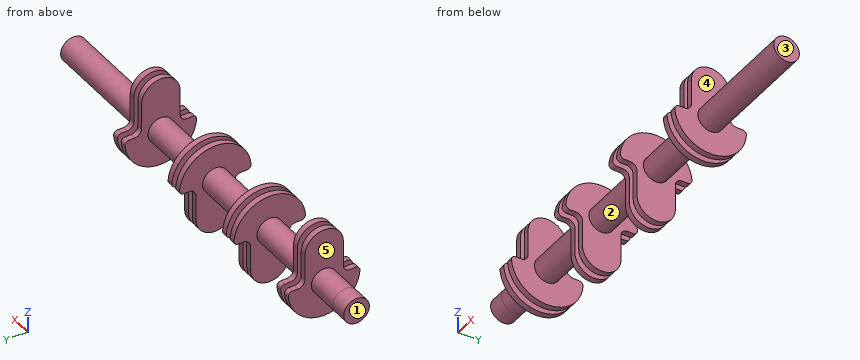
```python
from build123d import *

# Parameters (mm, degrees)
SKETCH1_R               = 15
BOSS_EXTRUDE1_DEPTH     = 400
BOSS_EXTRUDE2_START     = 53.5
BOSS_EXTRUDE2_DEPTH     = 7
BOSS_EXTRUDE3_START     = 39.5
BOSS_EXTRUDE3_DEPTH     = 7
BOSS_EXTRUDE4_START     = 339.5
BOSS_EXTRUDE4_DEPTH     = 7
BOSS_EXTRUDE5_START     = 353.5
BOSS_EXTRUDE5_DEPTH     = 7
CUT_EXTRUDE1_DEPTH      = 60
CUT_EXTRUDE1_DEPTH_BACK = 31
SKETCH5_W               = 7
SKETCH5_H               = 34.934316099
SKETCH5_H_2             = 32.180943616
BOSS_EXTRUDE6_START     = 46.5
SKETCH2_8_R             = 15
BOSS_EXTRUDE6_DEPTH     = 7
BOSS_EXTRUDE7_START     = 346.5
SKETCH2_9_R             = 15
BOSS_EXTRUDE7_DEPTH     = 7
BOSS_EXTRUDE8_START     = 139.5
BOSS_EXTRUDE8_DEPTH     = 7
BOSS_EXTRUDE9_START     = 153.5
BOSS_EXTRUDE9_DEPTH     = 7
BOSS_EXTRUDE10_START    = 239.5
BOSS_EXTRUDE10_DEPTH    = 7
BOSS_EXTRUDE11_START    = 253.5
BOSS_EXTRUDE11_DEPTH    = 7
CUT_EXTRUDE3_DEPTH      = 33
CUT_EXTRUDE3_DEPTH_BACK = 33
SKETCH8_W               = 7
SKETCH8_H               = 30
BOSS_EXTRUDE12_START    = 146.5
SKETCH6_6_R             = 15
BOSS_EXTRUDE12_DEPTH    = 7
BOSS_EXTRUDE13_START    = 246.5
SKETCH6_7_R             = 15
BOSS_EXTRUDE13_DEPTH    = 7
SKETCH9_R               = 15
BOSS_EXTRUDE14_DEPTH    = 100
SKETCH10_R              = 15
BOSS_EXTRUDE15_DEPTH    = 20


with BuildPart() as part:
    # Sketch1 → Boss-Extrude1 (new body)
    with BuildSketch(Plane(origin=(0, 0, 0), x_dir=(0, 0, -1), z_dir=(1, 0, 0))):
        Circle(SKETCH1_R)
    extrude(amount=BOSS_EXTRUDE1_DEPTH)

    # Sketch2 → Boss-Extrude2 (add)
    with BuildSketch(Plane.ZY.offset(-400).offset(BOSS_EXTRUDE2_START)):
        with BuildLine():
            Line((2, 30.5), (2, 37))
            ThreePointArc((2, 37), (0.389660992, 40.675622173), (-3.404079344, 41.983645241))
            ThreePointArc((-3.404079344, 41.983645241), (-42.121422387, 0), (-3.404079344, -41.983645241))
            ThreePointArc((-3.404079344, -41.983645241), (0.389660992, -40.675622173), (2, -37))
            Line((2, -37), (2, -30.5))
            ThreePointArc((2, -30.5), (4.343145751, -24.843145751), (10, -22.5))
            Line((10, -22.5), (40, -22.5))
            ThreePointArc((40, -22.5), (62.5, 0), (40, 22.5))
            Line((40, 22.5), (10, 22.5))
            ThreePointArc((10, 22.5), (4.343145751, 24.843145751), (2, 30.5))
        make_face()
    extrude(amount=BOSS_EXTRUDE2_DEPTH)

    # Sketch2_3 → Boss-Extrude3 (add)
    with BuildSketch(Plane.ZY.offset(-400).offset(BOSS_EXTRUDE3_START)):
        with BuildLine():
            Line((2, 30.5), (2, 37))
            ThreePointArc((2, 37), (0.389660992, 40.675622173), (-3.404079344, 41.983645241))
            ThreePointArc((-3.404079344, 41.983645241), (-42.121422387, 0), (-3.404079344, -41.983645241))
            ThreePointArc((-3.404079344, -41.983645241), (0.389660992, -40.675622173), (2, -37))
            Line((2, -37), (2, -30.5))
            ThreePointArc((2, -30.5), (4.343145751, -24.843145751), (10, -22.5))
            Line((10, -22.5), (40, -22.5))
            ThreePointArc((40, -22.5), (62.5, 0), (40, 22.5))
            Line((40, 22.5), (10, 22.5))
            ThreePointArc((10, 22.5), (4.343145751, 24.843145751), (2, 30.5))
        make_face()
    extrude(amount=BOSS_EXTRUDE3_DEPTH)

    # Sketch2_5 → Boss-Extrude4 (add)
    with BuildSketch(Plane.ZY.offset(-400).offset(BOSS_EXTRUDE4_START)):
        with BuildLine():
            Line((2, 30.5), (2, 37))
            ThreePointArc((2, 37), (0.389660992, 40.675622173), (-3.404079344, 41.983645241))
            ThreePointArc((-3.404079344, 41.983645241), (-42.121422387, 0), (-3.404079344, -41.983645241))
            ThreePointArc((-3.404079344, -41.983645241), (0.389660992, -40.675622173), (2, -37))
            Line((2, -37), (2, -30.5))
            ThreePointArc((2, -30.5), (4.343145751, -24.843145751), (10, -22.5))
            Line((10, -22.5), (40, -22.5))
            ThreePointArc((40, -22.5), (62.5, 0), (40, 22.5))
            Line((40, 22.5), (10, 22.5))
            ThreePointArc((10, 22.5), (4.343145751, 24.843145751), (2, 30.5))
        make_face()
    extrude(amount=BOSS_EXTRUDE4_DEPTH)

    # Sketch2_6 → Boss-Extrude5 (add)
    with BuildSketch(Plane.ZY.offset(-400).offset(BOSS_EXTRUDE5_START)):
        with BuildLine():
            Line((2, 30.5), (2, 37))
            ThreePointArc((2, 37), (0.389660992, 40.675622173), (-3.404079344, 41.983645241))
            ThreePointArc((-3.404079344, 41.983645241), (-42.121422387, 0), (-3.404079344, -41.983645241))
            ThreePointArc((-3.404079344, -41.983645241), (0.389660992, -40.675622173), (2, -37))
            Line((2, -37), (2, -30.5))
            ThreePointArc((2, -30.5), (4.343145751, -24.843145751), (10, -22.5))
            Line((10, -22.5), (40, -22.5))
            ThreePointArc((40, -22.5), (62.5, 0), (40, 22.5))
            Line((40, 22.5), (10, 22.5))
            ThreePointArc((10, 22.5), (4.343145751, 24.843145751), (2, 30.5))
        make_face()
    extrude(amount=BOSS_EXTRUDE5_DEPTH)

    # Sketch5 → Cut-Extrude1 (cut, two sides: drawn at the far end of the back side and taken through both)
    with BuildSketch(Plane(origin=(0, 0, 0), x_dir=(1, 0, 0), z_dir=(0, 1, 0)).offset(-CUT_EXTRUDE1_DEPTH_BACK)):
        with Locations((350, 2.467158049)):
            Rectangle(SKETCH5_W, SKETCH5_H)
        with Locations((50, 1.090471808)):
            Rectangle(SKETCH5_W, SKETCH5_H_2)
    extrude(amount=CUT_EXTRUDE1_DEPTH + CUT_EXTRUDE1_DEPTH_BACK, mode=Mode.SUBTRACT)


with BuildPart() as cut_extrude1_piece_1:
    # of the separate pieces the step leaves, piece 1, a body of its own (cut_extrude1_pieces)
    add(part.part.solids().sort_by_distance((53.5, 41.983645241, -3.404079344))[0])



with BuildPart() as cut_extrude1_piece_2:
    # of the separate pieces the step leaves, piece 2, a body of its own (cut_extrude1_pieces)
    add(part.part.solids().sort_by_distance((0, 0, -15))[0])


with BuildPart() as cut_extrude1_piece_3:
    # of the separate pieces the step leaves, piece 3, a body of its own (cut_extrude1_pieces)
    add(part.part.solids().sort_by_distance((353.5, 41.983645241, -3.404079344))[0])


with BuildPart() as cut_extrude1_piece_1_1:
    add(cut_extrude1_piece_1.part)

    add(cut_extrude1_piece_3.part)  # Boss-Extrude6 merges Cut-Extrude1 piece 3
    # Sketch2_8 → Boss-Extrude6 (add)
    with BuildSketch(Plane.ZY.offset(-400).offset(BOSS_EXTRUDE6_START)):
        with Locations((40, 0)):
            Circle(SKETCH2_8_R)
    extrude(amount=BOSS_EXTRUDE6_DEPTH)


    add(cut_extrude1_piece_2.part)  # Boss-Extrude7 merges Cut-Extrude1 piece 2
    # Sketch2_9 → Boss-Extrude7 (add)
    with BuildSketch(Plane.ZY.offset(-400).offset(BOSS_EXTRUDE7_START)):
        with Locations((40, 0)):
            Circle(SKETCH2_9_R)
    extrude(amount=BOSS_EXTRUDE7_DEPTH)

    # Sketch6 → Boss-Extrude8 (add)
    with BuildSketch(Plane(origin=(0, 0, 0), x_dir=(0, 0, -1), z_dir=(1, 0, 0)).offset(BOSS_EXTRUDE8_START)):
        with BuildLine():
            Line((2, 30.5), (2, 37))
            ThreePointArc((2, 37), (0.389660992, 40.675622173), (-3.404079344, 41.983645241))
            ThreePointArc((-3.404079344, 41.983645241), (-42.121422387, 0), (-3.404079344, -41.983645241))
            ThreePointArc((-3.404079344, -41.983645241), (0.389660992, -40.675622173), (2, -37))
            Line((2, -37), (2, -30.5))
            ThreePointArc((2, -30.5), (4.343145751, -24.843145751), (10, -22.5))
            Line((10, -22.5), (40, -22.5))
            ThreePointArc((40, -22.5), (62.5, 0), (40, 22.5))
            Line((40, 22.5), (10, 22.5))
            ThreePointArc((10, 22.5), (4.343145751, 24.843145751), (2, 30.5))
        make_face()
    extrude(amount=BOSS_EXTRUDE8_DEPTH)

    # Sketch6_3 → Boss-Extrude9 (add)
    with BuildSketch(Plane(origin=(0, 0, 0), x_dir=(0, 0, -1), z_dir=(1, 0, 0)).offset(BOSS_EXTRUDE9_START)):
        with BuildLine():
            Line((2, 30.5), (2, 37))
            ThreePointArc((2, 37), (0.389660992, 40.675622173), (-3.404079344, 41.983645241))
            ThreePointArc((-3.404079344, 41.983645241), (-42.121422387, 0), (-3.404079344, -41.983645241))
            ThreePointArc((-3.404079344, -41.983645241), (0.389660992, -40.675622173), (2, -37))
            Line((2, -37), (2, -30.5))
            ThreePointArc((2, -30.5), (4.343145751, -24.843145751), (10, -22.5))
            Line((10, -22.5), (40, -22.5))
            ThreePointArc((40, -22.5), (62.5, 0), (40, 22.5))
            Line((40, 22.5), (10, 22.5))
            ThreePointArc((10, 22.5), (4.343145751, 24.843145751), (2, 30.5))
        make_face()
    extrude(amount=BOSS_EXTRUDE9_DEPTH)

    # Sketch6_4 → Boss-Extrude10 (add)
    with BuildSketch(Plane(origin=(0, 0, 0), x_dir=(0, 0, -1), z_dir=(1, 0, 0)).offset(BOSS_EXTRUDE10_START)):
        with BuildLine():
            Line((2, 30.5), (2, 37))
            ThreePointArc((2, 37), (0.389660992, 40.675622173), (-3.404079344, 41.983645241))
            ThreePointArc((-3.404079344, 41.983645241), (-42.121422387, 0), (-3.404079344, -41.983645241))
            ThreePointArc((-3.404079344, -41.983645241), (0.389660992, -40.675622173), (2, -37))
            Line((2, -37), (2, -30.5))
            ThreePointArc((2, -30.5), (4.343145751, -24.843145751), (10, -22.5))
            Line((10, -22.5), (40, -22.5))
            ThreePointArc((40, -22.5), (62.5, 0), (40, 22.5))
            Line((40, 22.5), (10, 22.5))
            ThreePointArc((10, 22.5), (4.343145751, 24.843145751), (2, 30.5))
        make_face()
    extrude(amount=BOSS_EXTRUDE10_DEPTH)

    # Sketch6_5 → Boss-Extrude11 (add)
    with BuildSketch(Plane(origin=(0, 0, 0), x_dir=(0, 0, -1), z_dir=(1, 0, 0)).offset(BOSS_EXTRUDE11_START)):
        with BuildLine():
            Line((2, 30.5), (2, 37))
            ThreePointArc((2, 37), (0.389660992, 40.675622173), (-3.404079344, 41.983645241))
            ThreePointArc((-3.404079344, 41.983645241), (-42.121422387, 0), (-3.404079344, -41.983645241))
            ThreePointArc((-3.404079344, -41.983645241), (0.389660992, -40.675622173), (2, -37))
            Line((2, -37), (2, -30.5))
            ThreePointArc((2, -30.5), (4.343145751, -24.843145751), (10, -22.5))
            Line((10, -22.5), (40, -22.5))
            ThreePointArc((40, -22.5), (62.5, 0), (40, 22.5))
            Line((40, 22.5), (10, 22.5))
            ThreePointArc((10, 22.5), (4.343145751, 24.843145751), (2, 30.5))
        make_face()
    extrude(amount=BOSS_EXTRUDE11_DEPTH)

    # Sketch8 → Cut-Extrude3 (cut, two sides: drawn at the far end of the back side and taken through both)
    with BuildSketch(Plane(origin=(0, 0, 0), x_dir=(1, 0, 0), z_dir=(0, 1, 0)).offset(-CUT_EXTRUDE3_DEPTH_BACK)):
        with Locations((150, 0)):
            Rectangle(SKETCH8_W, SKETCH8_H)
        with Locations((250, 0)):
            Rectangle(SKETCH8_W, SKETCH8_H)
    extrude(amount=CUT_EXTRUDE3_DEPTH + CUT_EXTRUDE3_DEPTH_BACK, mode=Mode.SUBTRACT)


with BuildPart() as cut_extrude3_piece_1:
    # of the separate pieces the step leaves, piece 1, a body of its own (cut_extrude3_pieces)
    add(cut_extrude1_piece_1_1.part.solids().sort_by_distance((0, 0, -15))[0])



with BuildPart() as cut_extrude3_piece_2:
    # of the separate pieces the step leaves, piece 2, a body of its own (cut_extrude3_pieces)
    add(cut_extrude1_piece_1_1.part.solids().sort_by_distance((253.5, 22.5, -10))[0])


with BuildPart() as cut_extrude3_piece_3:
    # of the separate pieces the step leaves, piece 3, a body of its own (cut_extrude3_pieces)
    add(cut_extrude1_piece_1_1.part.solids().sort_by_distance((153.5, 22.5, -10))[0])


with BuildPart() as cut_extrude3_piece_1_1:
    add(cut_extrude3_piece_1.part)

    add(cut_extrude3_piece_3.part)  # Boss-Extrude12 merges Cut-Extrude3 piece 3
    # Sketch6_6 → Boss-Extrude12 (add)
    with BuildSketch(Plane(origin=(0, 0, 0), x_dir=(0, 0, -1), z_dir=(1, 0, 0)).offset(BOSS_EXTRUDE12_START)):
        with Locations((40, 0)):
            Circle(SKETCH6_6_R)
    extrude(amount=BOSS_EXTRUDE12_DEPTH)


    add(cut_extrude3_piece_2.part)  # Boss-Extrude13 merges Cut-Extrude3 piece 2
    # Sketch6_7 → Boss-Extrude13 (add)
    with BuildSketch(Plane(origin=(0, 0, 0), x_dir=(0, 0, -1), z_dir=(1, 0, 0)).offset(BOSS_EXTRUDE13_START)):
        with Locations((40, 0)):
            Circle(SKETCH6_7_R)
    extrude(amount=BOSS_EXTRUDE13_DEPTH)

    # Sketch9 → Boss-Extrude14 (add)
    with BuildSketch(Plane(origin=(400, 0, 0), x_dir=(0, 0, -1), z_dir=(1, 0, 0))):
        with Locations(Location((0, 0, 0), (0, 0, 180))):
            Circle(SKETCH9_R)
    extrude(amount=BOSS_EXTRUDE14_DEPTH)

    # Sketch10 → Boss-Extrude15 (add)
    with BuildSketch(Plane.ZY):
        Circle(SKETCH10_R)
    extrude(amount=BOSS_EXTRUDE15_DEPTH)


solid = cut_extrude3_piece_1_1.part
```
The model under review builds one solid part; all positions refer to its coordinate system, in mm. Face numbers are marked on the shaded views. A direction names the side the tool comes from. Round coordinates to 2 decimals unless told otherwise and drop trailing zeros. Write each loop counter-clockwise with the first axis right and the second up, starting at its lowest first coordinate (ties: lowest second). Pieces come first, ordered by that corner, then holes. Notation, with made-up numbers: (-10.75, -36) - (9.25, -36) arc R18 cw to (9.25, -1) - close; hole circle Ø10 at (27, 39.5). An arc over 180 degrees is marked (long way). One line per question, with ' | ' between items.
Item 1: For P1, Ø7.5, axis at x = 341.5, z = 27, coming from the +Y side; P2, Ø12, axis at x = 255.5, z = -18.5, coming from the -Y side; P3, Ø7, axis at x = 142, y = 33, coming from the -Z side, all flat-tipped, find the tip position at first contact; note any pin that passes through.
Resolved:
P1: stops at y = 22.5 | P2: stops at y = -22.5 | P3: stops at z = -2.06
Item 2: Add section B-B, the plane x = 310. Give the boundary of the cut face in (y, z).
Resolved:
outline: circle Ø30 at (0, 0)
Item 3: To check wall thickness, follow probe 1 along X at (y, z) = (7.5, 30); probe 2 along X at (y, z) = (6.5, -0.5); probe 3 along X at (y, z) = (-23, 15.5). State the ranges of each line that lie inside material, in increasing order.
Resolved:
probe 1: x = 39.5 to 60.5, 139.5 to 146.5, 153.5 to 160.5, 239.5 to 246.5, 253.5 to 260.5, 339.5 to 360.5 | probe 2: x = -20 to 46.5, 53.5 to 146.5, 153.5 to 246.5, 253.5 to 346.5, 353.5 to 500 | probe 3: x = 139.5 to 146.5, 153.5 to 160.5, 239.5 to 246.5, 253.5 to 260.5
Item 4: For the marked faces 1, 2, 3, 4 and 5, list the 3-axis set-ups (+Z, -Z, +X, -X, +Y, -Y) from which the entire face can be reached by the end or side of a thin tool; tool diameter is ignored.
Resolved:
face 1: +Z, -Z, -X, +Y, -Y | face 2: none | face 3: +Z, -Z, +X, +Y, -Y | face 4: +X | face 5: -X
Item 5: Add section A-A, the plane z = -47. Give the boundary of the cut face in (x, y), then the cut area to 3 significant figures.
Resolved:
outline: (139.5, -21.38) - (146.5, -21.38) - (146.5, -13.27) - (153.5, -13.27) - (153.5, -21.38) - (160.5, -21.38) - (160.5, 21.38) - (153.5, 21.38) - (153.5, 13.27) - (146.5, 13.27) - (146.5, 21.38) - (139.5, 21.38) - close; (239.5, -21.38) - (246.5, -21.38) - (246.5, -13.27) - (253.5, -13.27) - (253.5, -21.38) - (260.5, -21.38) - (260.5, 21.38) - (253.5, 21.38) - (253.5, 13.27) - (246.5, 13.27) - (246.5, 21.38) - (239.5, 21.38) - close | area: 1,570 mm2
